The model under review builds one solid part; all positions refer to its coordinate system, in mm. A direction names the side the tool comes from. Round coordinates to 2 decimals unless told otherwise and drop trailing zeros. Write each loop counter-clockwise with the first axis right and the second up, starting at its lowest first coordinate (ties: lowest second). Pieces come first, ordered by that corner, then holes.
Item 1: Add section C-C (y = -39). Give the boundary of the cut face in (x, z) (3 decimals), plus the area to 3 significant figures.
Item 2: Add section B-B (x = -20). Give the boundary of the cut face in (y, z) (3 decimals), plus the area to 3 significant figures.
Item 3: Clearance check with a flat-ended pin moving along its axis: pin 1 Ø1 at (x, y) = (29.5, -10.5) entering from +Z. State where the tip first meets the part, or that it passes through.
Item 4: Add section A-A (z = 14.5). Give the boundary of the cut face in (x, y) (3 decimals), plus the area to 3 significant figures.
Item 5: Machinability: for faces 5 (the face through (38.1, -1, 20)), 6 (the face through (-1, 54.61, 13)), which of the approach directions +Z, -Z, +X, -X, +Y, -Y give a long, thin tool a straight path to every point of the face, cutting with its end or side? Answer none if there is none.
Item 6: To check wall thickness, follow L1, parallel to Y at x = 9.5, z = 13.25 (3 decimals); L2, parallel to Y at x = -17, z = 23; L3, parallel to X at y = -26, z = 18.75. State the ranges of each line that lie inside material, in increasing order.
Item 7: Draft analysis for pull direction X (two halves, no side actions). For faces 1 (the face through (41.91, -1, 13)), 2 (the face through (-34, 3, 12.7)), 3 (the face through (33.655, -1, 15)), 4 (the face through (-1, -54.61, 13)), state which applies: +X half, -X half, draft (parallel to the pull), parting line (faces both ways), or undercut.
```python
from build123d import *

# Parameters (mm, degrees)
F0_W     = 76.2
F0_H     = 101.6
F1_DEPTH = 12.7
F0_W_2   = 83.82
F0_H_2   = 109.22
F2_DEPTH = 25.4
F3_W     = 67.31
F3_H     = 92.71
F4_DEPTH = 5.08
F5_W     = 76.2
F5_H     = 2.54
F6_DEPTH = 5.08


with BuildPart() as f1:
    # F0 (on Top) → F1 (new body)
    with BuildSketch(Plane.XY):
        Rectangle(F0_W, F0_H)
    extrude(amount=F1_DEPTH)

    # F0 (on Top) → F2 (join)
    with BuildSketch(Plane.XY):
        Rectangle(F0_W_2, F0_H_2)
        Rectangle(F0_W, F0_H, mode=Mode.SUBTRACT)
    extrude(amount=F2_DEPTH)

    # F3 (on face) → F4 (join)
    with BuildSketch(Plane.XY.offset(12.7)):
        Rectangle(F3_W, F3_H)
    extrude(amount=F4_DEPTH)

    # F5 (on face) → F6 (cut)
    with BuildSketch(Plane.XY.offset(12.7)):
        with Locations((0, 49.53)):
            Rectangle(F5_W, F5_H)
    extrude(amount=-F6_DEPTH, mode=Mode.SUBTRACT)


solid = f1.part
```
Numbers:
1. outline: (-41.91, 0) - (41.91, 0) - (41.91, 25.4) - (38.1, 25.4) - (38.1, 12.7) - (33.655, 12.7) - (33.655, 17.78) - (-33.655, 17.78) - (-33.655, 12.7) - (-38.1, 12.7) - (-38.1, 25.4) - (-41.91, 25.4) - close
1. area: 1,500 mm2
2. outline: (-54.61, 0) - (54.61, 0) - (54.61, 25.4) - (50.8, 25.4) - (50.8, 7.62) - (48.26, 7.62) - (48.26, 12.7) - (46.355, 12.7) - (46.355, 17.78) - (-46.355, 17.78) - (-46.355, 12.7) - (-50.8, 12.7) - (-50.8, 25.4) - (-54.61, 25.4) - close
2. area: 1,940 mm2
3. pin 1: stops at z = 17.78
4. outline: (-41.91, -54.61) - (41.91, -54.61) - (41.91, 54.61) - (-41.91, 54.61) - close; (-33.655, -46.355) - (33.655, -46.355) - (33.655, 46.355) - (-33.655, 46.355) - close; hole (-38.1, -50.8) - (38.1, -50.8) - (38.1, 50.8) - (-38.1, 50.8) - close
4. area: 7,650 mm2
5. face 5: +Z
5. face 6: +Z, -Z, +X, -X, +Y
6. L1: y = -54.61 to -50.8, -46.355 to 46.355, 50.8 to 54.61
6. L2: y = -54.61 to -50.8, 50.8 to 54.61
6. L3: x = -41.91 to -38.1, 38.1 to 41.91
7. face 1: +X half
7. face 2: undercut
7. face 3: undercut
7. face 4: draft
